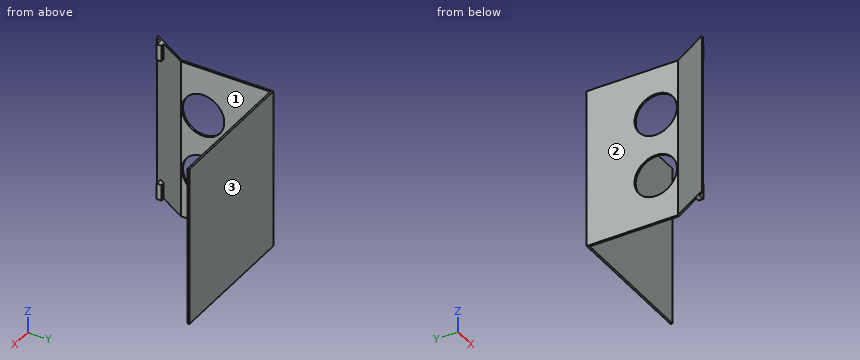
```python
from build123d import *

# Parameters (mm, degrees)
SALIENTE_EXTRUIR1_DEPTH = 100
SALIENTE_EXTRUIR2_DEPTH = 10
SALIENTE_EXTRUIR3_DEPTH = 10
CROQUIS9_R              = 13.25
CORTAR_EXTRUIR5_DEPTH   = 10


with BuildPart() as part:
    # Croquis1 → Saliente-Extruir1 (new body)
    with BuildSketch(Plane.XY):
        Polygon((0, 0), (1.2, 0), (14.45, 22.9496732), (14.45, 78.7596732), (100, 78.7596732), (100, 79.9596732), (13.25, 79.9596732), (13.25, 22.9496732), align=None)
    extrude(amount=-SALIENTE_EXTRUIR1_DEPTH)

    # Croquis2 → Saliente-Extruir2 (add)
    with BuildSketch(Plane.XY):
        Polygon((3.162990915, 3.4), (7.162990915, 3.4), (7.162990915, 6.4), (4.895041723, 6.4), align=None)
    extrude(amount=-SALIENTE_EXTRUIR2_DEPTH)

    # Croquis4 → Saliente-Extruir3 (add)
    with BuildSketch(Plane(origin=(0, 0, -100), x_dir=(-1, 0, 0), z_dir=(0, 0, -1))):
        Polygon((-3.162990915, 3.4), (-7.162990915, 3.4), (-7.162990915, 6.4), (-4.895041723, 6.4), align=None)
    extrude(amount=-SALIENTE_EXTRUIR3_DEPTH)

    # Croquis9 → Cortar-Extruir5 (cut)
    with BuildSketch(Plane.ZY.offset(-13.25)):
        with BuildLine():
            ThreePointArc((-56.35, 36.8), (-78.969164851, 46.169164851), (-69.6, 23.55))
            Line((-69.6, 23.55), (-69.6, 36.8))
            Line((-69.6, 36.8), (-56.35, 36.8))
        make_face()
        with BuildLine():
            Line((-69.6, 36.8), (-69.6, 23.55))
            ThreePointArc((-69.6, 23.55), (-60.230835149, 27.430835149), (-56.35, 36.8))
            Line((-56.35, 36.8), (-69.6, 36.8))
        make_face()
        with Locations(Location((-30.07, 36.8, 0), (0, 0, 270))):
            Circle(CROQUIS9_R)
    extrude(amount=-CORTAR_EXTRUIR5_DEPTH, mode=Mode.SUBTRACT)


solid = part.part
```
The model under review builds one solid part; all positions refer to its coordinate system, in mm. Face numbers are marked on the shaded views. A direction names the side the tool comes from. Round coordinates to 2 decimals unless told otherwise and drop trailing zeros. Order: outer loops, then holes, each group sorted by start corner. A loop starts at its lowest first (then second) coordinate and runs counter-clockwise, first axis right, second up. Notation, with made-up numbers: M -35,29.5 L 10,29.5 A8 ccw 10,42.5 Z; hole C -8,48 d10. An arc over 180 degrees is marked long. Use a Markdown table: item, result.
1) Consider section B-B (y = 40). Write out the cut boundary in (x, z), then the cut area to 3 significant figures.
Report:
| item | result |
|---|---|
| outline | M 13.25,-100 L 14.45,-100 L 14.45,-82.46 L 13.25,-82.46 Z; M 13.25,-56.74 L 14.45,-56.74 L 14.45,-42.93 L 13.25,-42.93 Z; M 13.25,-17.21 L 14.45,-17.21 L 14.45,0 L 13.25,0 Z |
| area | 58.3 mm^2 |
2) Insertion check: pin 1 (10 mm diameter, centred on y = 68.5, z = -69.5, fed in from +X); pin 2 (0.7 mm diameter, centred on x = 5.5, z = -97.5, fed in from +Y); pin 3 (0.9 mm diameter, centred on x = 5, y = 4.5, fed in from +Z); pin 4 (10 mm diameter, centred on y = 42.5, z = -15.5, fed in from -X). Each pin has a flat end and moves straight along its axis. Give the tip position at first contact, or say it passes through.
Report:
| item | result |
|---|---|
| pin 1 | x = 14.45 |
| pin 2 | y = 10.13 |
| pin 3 | z = 0 |
| pin 4 | x = 13.25 |
3) Consider section C-C (z = -52). Write out the cut boundary in (x, y), then the cut area to 3 significant figures.
Report:
| item | result |
|---|---|
| outline | M 0,0 L 1.2,0 L 14.45,22.95 L 14.45,78.76 L 100,78.76 L 100,79.96 L 13.25,79.96 L 13.25,22.95 Z |
| area | 199 mm^2 |
4) Wall thickness on line 1 along Z through (x, y) = (14, 36.8); line 2 along Y through (x, z) = (42.5, -40); line 3 along X through (y, z) = (53, -82.5): over which ranges is each line inside the solid? List them lowest first. Write a range as [from, to].
Report:
| item | result |
|---|---|
| line 1 | [-100, -82.85], [-56.35, -43.32], [-16.82, 0] |
| line 2 | [78.76, 79.96] |
| line 3 | [13.25, 14.45] |
5) Tool access review of the marked faces 1, 2 and 3: name each direction out of +Z, -Z, +X, -X, +Y, -Y from which nothing blocks a thin tool from reaching the whole face with its end or side.
Report:
| item | result |
|---|---|
| face 1 | +Z, -Z, +X, -Y |
| face 2 | +Z, -Z, -X, +Y |
| face 3 | +Z, -Z, +X, -X, +Y |
6) Consider section A-A (z = -30.07). Write out the cut boundary in (x, y).
Report:
| item | result |
|---|---|
| outline | M 0,0 L 1.2,0 L 14.45,22.95 L 14.45,23.55 L 13.25,23.55 L 13.25,22.95 Z; M 13.25,50.05 L 14.45,50.05 L 14.45,78.76 L 100,78.76 L 100,79.96 L 13.25,79.96 Z |
7) Consider section D-D (x = 78.5). Write out the cut boundary in (y, z).
Report:
| item | result |
|---|---|
| outline | M 78.76,-100 L 79.96,-100 L 79.96,0 L 78.76,0 Z |
